```python
from build123d import *

# Parameters (mm, degrees)
PAD002_DEPTH  = 50
CHAMFER_SIZE2 = 125
CHAMFER_SIZE  = 49
FILLET_R      = 80


with BuildPart() as part:
    # Sketch004 → Pad002 (new body, symmetric)
    with BuildSketch(Plane.XZ):
        Polygon((0, 0), (300, 0), (300, 550), (50, 550), align=None)
    extrude(amount=PAD002_DEPTH, both=True)

    # Chamfer
    chamfer_edges = [part.edges().sort_by_distance(p)[0] for p in [
        (25, 50, 275),
        (25, -50, 275),
    ]]
    chamfer_side = part.faces().sort_by_distance((25, 0, 275))[0]
    chamfer(chamfer_edges, length=CHAMFER_SIZE, length2=CHAMFER_SIZE2, reference=chamfer_side)


with BuildPart() as part_1:
    # Body005 placement: moved
    add(part.part.moved(Location((3844.9642, 0, 513))))

    # Fillet
    fillet_edges = [part_1.edges().sort_by_distance(p)[0] for p in [
        (3995.479666, 50, 788),
        (3995.479666, -50, 788),
    ]]
    fillet(fillet_edges, radius=FILLET_R)


solid = part_1.part
```
The model under review builds one solid part; all positions refer to its coordinate system, in mm. A direction names the side the tool comes from. Give positions to 0.01 mm unless a question says otherwise; leave off trailing zeros. Write each loop counter-clockwise with the first axis right and the second up, starting at its lowest first coordinate (ties: lowest second). Pieces come first, ordered by that corner, then holes. Notation, with made-up numbers: M 50.25,81 L 79.25,81 A22 ccw 79.25,113 Z; hole C 0,-12.75 d6. An arc over 180 degrees is marked long. Write item = value, one per line. Start each with the question number.
Q1. We need section A-A (x = 3922.5). State the section outline as (y, z) points, plus the area to 3 significant figures.
Q2. Machinability: for faces 1 (the face through (4082, 50, 792)), 2 (the face through (3995.599, -48.647, 784.136)), 3 (the face through (3995.599, 48.647, 784.136)), which of the approach directions +Z, -Z, +X, -X, +Y, -Y give a long, thin tool a straight path to every point of the face, cutting with its end or side? Answer none if there is none.
Q3. We need section B-B (y = -11). State the section outline as (x, z) points.
Q4. For line 1 (Y direction, x = 3871.5, z = 797.5); line 2 (Y direction, x = 3888, z = 582); line 3 (X direction, y = 0, z = 763.5), list the stretches that pass through material, from the lowest coordinate up.
Q5. Clearance check with flat-ended pins moving along their axes: pin 1 (5 mm diameter, centred on x = 3931, z = 668, fed in from -Y); pin 2 (3 mm diameter, centred on x = 3932, z = 985, fed in from +Y); pin 3 (10 mm diameter, centred on x = 4012, z = 970.5, fed in from -Y). State where each tip first meets the part, or that it passes through.
Result set:
q1.outline = M -31.27,513 L 31.27,513 L 11.75,1063 L -11.75,1063 Z
q1.area = 23,700 mm2
q2.face_1 = +Z, -Z, +X, -X, +Y
q2.face_2 = +Z, -X, -Y
q2.face_3 = +Z, -X, +Y
q3.outline = M 3870.58,513 L 4144.96,513 L 4144.96,1063 L 3920.58,1063 Z
q4.line_1 = -1.26 to 1.26
q4.line_2 = -15.35 to 15.35
q4.line_3 = 3867.74 to 4144.96
q5.pin_1 = -30.07
q5.pin_2 = 18.81
q5.pin_3 = -49.35
